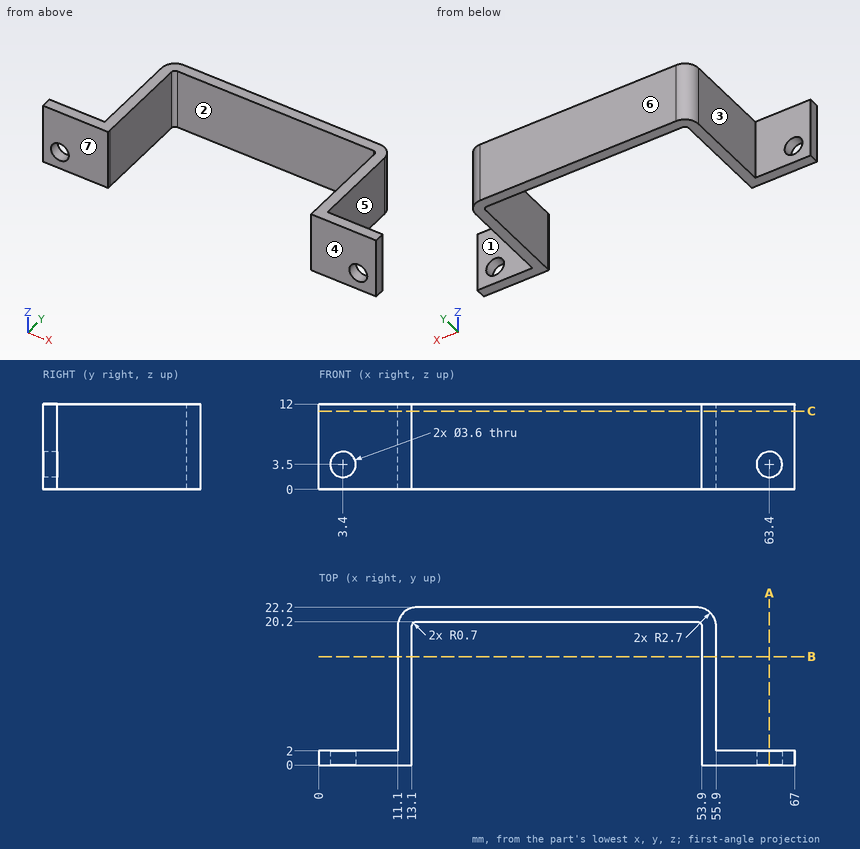
Job drawing, mm, ordinate dimensions from the low corner. One solid piece. A direction names the side the tool comes from. Round coordinates to 2 decimals unless told otherwise and drop trailing zeros. Loops run counter-clockwise (first coordinate to the right, second up) from the corner with the lowest first, then second, coordinate; pieces in that order, holes last.
Item 1: Mould opens along Y. For the marked faces 5, 6 and 7 say: +Y half, -Y half, draft (parallel to the pull), parting line (faces both ways), or undercut.
Item 2: Drop flat-ended pins along their axis: P1, Ø6, axis at x = 63.4, z = 3.5, coming from the +Y side; P2, Ø6, axis at x = 34, z = 8.5, coming from the -Y side; P3, Ø6, axis at y = 12, z = 7.5, coming from the +X side; P4, Ø2, axis at x = 3.4, z = 3.5, coming from the +Y side. Give the stop position or say it passes through.
Item 3: Cut at A-A, the plane x = 63.4. Give the cut face in (y, z).
Item 4: Drill centre lines: line 1 (Z direction, x = 63.4, y = 1.1); line 2 (X direction, y = 15, z = 7.25); line 3 (Y direction, x = 56, z = 4.75). Where is each one in solid material? Low to high.
Item 5: Cut at C-C, the plane z = 11. Give the cut face in (x, y), then the cut area to 3 significant figures.
Item 6: Cut at B-B, the plane y = 15.25. Give the cut face in (x, z), then the cut area to 3 significant figures.
Item 7: 3-axis set-ups, long thin cutter, end or side, ignore diameter. For the marked faces 1, 2, 3 and 4: which of +Z, -Z, +X, -X, +Y, -Y reach the whole face in a straight line?
A:
1. face 5: draft
1. face 6: +Y half
1. face 7: -Y half
2. P1: stops at y = 2
2. P2: stops at y = 20.2
2. P3: stops at x = 55.9
2. P4: passes through
3. outline: (0, 0) - (2, 0) - (2, 1.7) - (0, 1.7) - close; (0, 5.3) - (2, 5.3) - (2, 12) - (0, 12) - close
4. line 1: z = 0 to 1.7, 5.3 to 12
4. line 2: x = 11.1 to 13.1, 53.9 to 55.9
4. line 3: y = 0 to 2
5. outline: (0, 0) - (13.1, 0) - (13.1, 19.5) arc R0.7 cw to (13.8, 20.2) - (53.2, 20.2) arc R0.7 cw to (53.9, 19.5) - (53.9, 0) - (67, 0) - (67, 2) - (55.9, 2) - (55.9, 19.5) arc R2.7 ccw to (53.2, 22.2) - (13.8, 22.2) arc R2.7 ccw to (11.1, 19.5) - (11.1, 2) - (0, 2) - close
5. area: 212 mm2
6. outline: (11.1, 0) - (13.1, 0) - (13.1, 12) - (11.1, 12) - close; (53.9, 0) - (55.9, 0) - (55.9, 12) - (53.9, 12) - close
6. area: 48.0 mm2
7. face 1: +Z, -Z, +X, +Y
7. face 2: +Z, -Z, -Y
7. face 3: +Z, -Z, -X, +Y
7. face 4: +Z, -Z, +X, -X, -Y
